Design review of the part built by this model. Coordinates are the model's own, in mm. A direction names the side the tool comes from. Give positions to 0.01 mm unless a question says otherwise; leave off trailing zeros. Loops run counter-clockwise (first coordinate to the right, second up) from the corner with the lowest first, then second, coordinate; pieces in that order, holes last. Notation, with made-up numbers: (-14, 88) - (6, 88) arc R24 ccw to (6, 127) - close; hole circle Ø8 at (49, 6). An arc over 180 degrees is marked (long way). Write each question's results on one line, items separated by ' | '.
Autodesk Inventor part; units mm, degrees
ref_plane "YZ Plane" through (0, 0, 0) normal (1, 0, 0) x (0, 1, 0)
ref_plane "XZ Plane" through (0, 0, 0) normal (0, 1, 0) x (-1, 0, 0)
ref_plane "XY Plane" through (0, 0, 0) normal (0, 0, 1) x (1, 0, 0)
sketch "Skizze1" plane through (0, 0, 0) normal (0, 0, 1) x (1, 0, 0)
  circle A0 centre (0, 0) radius 2.5
  dimension "d0" = 5
extrude "Extrusion1" add sketch "Skizze1" along normal blind 8.5
fillet "Rundung1" radius 2.5 1 edges at (-2.5, 0, 8.5)
sketch "Skizze2" plane through (0, 0, 0) normal (0, 0, -1) x (-1, 0, 0)
  circle A0 centre (0, 0) radius 2.5
  circle A1 centre (0, 0) radius 3
  dimension "d4" = 6
extrude "Extrusion2" add sketch "Skizze2" against normal blind 1
sketch "Skizze3" plane through (0, 0, 0) normal (0, 0, -1) x (-1, 0, 0)
  circle A0 centre (0, 0) radius 3
  circle A1 centre (0, 2) radius 0.5
  circle A2 centre (0, -2) radius 0.5
  point P0 (0, 3)
  point P1 (0, -3)
  dimension "d7" = 1
  dimension "d8" = 1
  dimension "d9" = 1
  dimension "d10" = 1
extrude "Extrusion3" add sketch "Skizze3" along normal blind 28 contours A1 | A2
properties part number "LED´s"
Item 1: We need section C-C on z = 3. Give the boundary of the cut face in (x, y).
Output values:
outline: circle Ø5 at (0, 0)
Item 2: We need section A-A on x = 0. Give the boundary of the cut face in (y, z).
Output values:
outline: (-3, 0) - (-2.5, 0) - (-2.5, -28) - (-1.5, -28) - (-1.5, 0) - (1.5, 0) - (1.5, -28) - (2.5, -28) - (2.5, 0) - (3, 0) - (3, 1) - (2.5, 1) - (2.5, 6) arc R2.5 ccw to (-2.5, 6) - (-2.5, 1) - (-3, 1) - close
Item 3: We need section B-B on y = 0. Give the boundary of the cut face in (x, z), then the cut area to 3 significant figures.
Output values:
outline: (-3, 0) - (3, 0) - (3, 1) - (2.5, 1) - (2.5, 6) arc R2.5 ccw to (-2.5, 6) - (-2.5, 1) - (-3, 1) - close | area: 40.8 mm²
Item 4: We need section D-D on z = -8.5. Give the boundary of the cut face in (x, y), then the cut area to 3 significant figures.
Output values:
outline: circle Ø1 at (0, -2); circle Ø1 at (0, 2) | area: 1.57 mm²
Item 5: Clearance check with flat-ended pins moving along their axes: P1, Ø1, axis at x = 0, y = 1.5, coming from the +Z side; P2, Ø3, axis at x = 2, y = -1, coming from the +Z side. State where each tip first meets the part, or that it passes through.
Output values:
P1: stops at z = 8.29 | P2: stops at z = 8.39
Item 6: Draft analysis for pull direction Y (two halves, no side actions). For faces 4 (the face through (0, -2, -28)), 5 (the face through (0.065, -2.496, -13.804)), 6 (the face through (-0.54, 2.44, 3.46)), state which applies: +Y half, -Y half, draft (parallel to the pull), parting line (faces both ways), or undercut.
Output values:
face 4: draft | face 5: undercut | face 6: parting line
Item 7: Wall thickness on probe 1 along X at (y, z) = (-1.95, -15); probe 2 along Z at (x, y) = (2.35, -1.55); probe 3 along Y at (x, z) = (-0.2, 6): over which ranges is each line inside the solid? List them lowest first.
Output values:
probe 1: x = -0.5 to 0.5 | probe 2: z = 0 to 1 | probe 3: y = -2.49 to 2.49
Item 8: Tool access review of faces 1 (the face through (3, 0.1, 0.5)), 2 (the face through (0.065, 1.504, -13.804)), 3 (the face through (2, 2, 1)): name each direction out of +Z, -Z, +X, -X, +Y, -Y from which nothing blocks a thin tool from reaching the whole face with its end or side.
Output values:
face 1: +Z, -Z | face 2: -Z | face 3: +Z
